from build123d import *

# Parameters (mm, degrees)
SKETCH_3_W          = 180
SKETCH_3_H          = 43
EXTRUDE_1_DEPTH     = 12
CUT_EXTRUDE_1_DEPTH = 52
CUT_EXTRUDE_2_DEPTH = 5
CUT_EXTRUDE_3_DEPTH = 5
SKETCH_8_W          = 55
SKETCH_8_H          = 37
CUT_EXTRUDE_4_DEPTH = 10.5
CUT_EXTRUDE_5_DEPTH = 3
SKETCH_10_W         = 62.128790526
SKETCH_10_H         = 8.683746703
CUT_EXTRUDE_6_DEPTH = 8
CUT_EXTRUDE_8_DEPTH = 9
FILLET_3_R          = 3
FILLET_4_R          = 2.5


with BuildPart() as part:
    # 草图3 → 凸台-拉伸1 (new body)
    with BuildSketch(Plane(origin=(0, 0, 0), x_dir=(1, 0, 0), z_dir=(0, 1, 0))):
        with Locations((50.068597249, 7.753123643)):
            Rectangle(SKETCH_3_W, SKETCH_3_H)
    extrude(amount=EXTRUDE_1_DEPTH)

    # 草图4 → 切除-拉伸1 (cut)
    with BuildSketch(Plane(origin=(0, 0, 0), x_dir=(1, 0, 0), z_dir=(0, 1, 0))):
        Polygon((-22.469613434, -5.858946979), (26.002261286, -5.858946979), (29.068597249, -13.746876357), (-25.931402751, -13.746876357), align=None)
    extrude(amount=CUT_EXTRUDE_1_DEPTH, mode=Mode.SUBTRACT)

    # 草图5 → 切除-拉伸2 (cut)
    with BuildSketch(Plane(origin=(0, 12, 0), x_dir=(1, 0, 0), z_dir=(0, 1, 0))):
        Polygon((140.068597249, 7.753123643), (140.068597249, 22.753123643), (125.276479966, 22.753123643), (125.276479966, -7.246876357), (140.068597249, -7.246876357), align=None)
    extrude(amount=-CUT_EXTRUDE_2_DEPTH, mode=Mode.SUBTRACT)

    # 草图7 → 切除-拉伸3 (cut)
    with BuildSketch(Plane(origin=(0, 12, 0), x_dir=(1, 0, 0), z_dir=(0, 1, 0))):
        Polygon((125.276479966, 7.753123643), (125.276479966, 25.753123643), (100.500825538, 25.753123643), (100.500825538, -10.246876357), (125.276479966, -10.246876357), align=None)
    extrude(amount=-CUT_EXTRUDE_3_DEPTH, mode=Mode.SUBTRACT)

    # 草图8 → 切除-拉伸4 (cut)
    with BuildSketch(Plane(origin=(0, 12, 0), x_dir=(1, 0, 0), z_dir=(0, 1, 0))):
        with Locations((63.776287419, 7.753123643)):
            Rectangle(SKETCH_8_W, SKETCH_8_H)
    extrude(amount=-CUT_EXTRUDE_4_DEPTH, mode=Mode.SUBTRACT)

    # 草图9 → 切除-拉伸5 (cut)
    with BuildSketch(Plane(origin=(0, 12, 0), x_dir=(1, 0, 0), z_dir=(0, 1, 0))):
        Polygon((91.276287419, 26.253123643), (96.635770173, 26.253123643), (96.635770173, 22.130591531), (96.635770173, 13.862098754), (97.813575381, 11.877191358), (100.500825538, 11.877191358), (100.500825538, 3.393971617), (96.236747254, 3.393971617), (92.132656028, 10.310430274), (92.132656028, 21.255120764), (91.276287419, 21.255120764), align=None)
    extrude(amount=-CUT_EXTRUDE_5_DEPTH, mode=Mode.SUBTRACT)

    # 草图10 → 切除-拉伸6 (cut)
    with BuildSketch(Plane(origin=(0, 12, 0), x_dir=(1, 0, 0), z_dir=(0, 1, 0))):
        with Locations((1.934159822, -6.405003006)):
            Rectangle(SKETCH_10_W, SKETCH_10_H)
    extrude(amount=-CUT_EXTRUDE_6_DEPTH, mode=Mode.SUBTRACT)

    # 草图11 → 切除-拉伸8 (cut)
    with BuildSketch(Plane(origin=(0, 12, 0), x_dir=(1, 0, 0), z_dir=(0, 1, 0))):
        Polygon((32.998555085, -10.746876357), (-36.5396752, -10.746876357), (-36.5396752, 26.253123643), (36.276287419, 26.253123643), (36.276287419, -2.167243749), (32.998555085, -2.063129654), align=None)
    extrude(amount=-CUT_EXTRUDE_8_DEPTH, mode=Mode.SUBTRACT)

    # 圆角3
    fillet_3_edges = [part.edges().sort_by_distance(p)[0] for p in [
        (-39.931402751, 6, -29.253123643),
        (140.068597249, 6, -29.253123643),
        (140.068597249, 6, 13.746876357),
        (-39.931402751, 6, 13.746876357),
    ]]
    fillet(fillet_3_edges, radius=FILLET_3_R)

    # 圆角4
    fillet_4_edges = [part.edges().sort_by_distance(p)[0] for p in [
        (83.068597249, 0, 13.746876357),
        (50.068597249, 0, -29.253123643),
        (-31.431402751, 0, 13.746876357),
        (-39.931402751, 0, -7.753123643),
        (140.068597249, 0, -7.753123643),
        (-39.052723094, 0, -28.374443987),
        (-39.052723094, 0, 12.8681967),
        (139.189917593, 0, 12.8681967),
        (139.189917593, 0, -28.374443987),
    ]]
    fillet(fillet_4_edges, radius=FILLET_4_R)


solid = part.part
Verification items for the finished model (mm, model axes). A direction names the side the tool comes from. Give positions to 0.01 mm unless a question says otherwise; leave off trailing zeros. Loops run counter-clockwise (first coordinate to the right, second up) from the corner with the lowest first, then second, coordinate; pieces in that order, holes last.
1) Depth check by flat-ended pin: pin 1 Ø8 at (x, z) = (25.5, 6) entering from -Y; pin 2 Ø1 at (x, y) = (22, 2.5) entering from +Z; pin 3 Ø5.5 at (y, z) = (10.5, -4.5) entering from +X; pin 4 Ø8 at (x, z) = (73.5, -13) entering from +Y. Enter the tip coordinate at first touch or a pass-through.
2) Sectioned sample at D-D, the plane x = -2.5. Enter the section's corners in (y, z).
3) Set-up check for faces 1 (the flat face through (28.195, 4.583, 11.501)), 2 (the flat face through (29, 7, -26.253)), 3 (the flat face through (94.213, 10.521, -6.804)): record each of +Z, -Z, +X, -X, +Y, -Y from which the full face is reachable in a straight line by a thin tool's end or side.
4) Sectioned sample at C-C, the plane x = 116.5. Enter the section's corners in (y, z), then the cut area to 3 significant figures.
5) Draft check along Z on faces 4 (the flat face through (125.276, 10, -24)), 5 (the cylindrical face through (-39.076, 7.316, -28.351)), 6 (the flat face through (23, 12, -27)). Enter one of: pulls with the +Z half, pulls with the -Z half, needs draft (parallel to the pull), parting line crosses it, or undercut.
6) Sectioned sample at A-A, the plane x = 81. Enter the section's corners in (y, z).
7) Sectioned sample at B-B, the plane z = -8. Enter the section's corners in (x, y), then the cut area to 3 significant figures.
8) Thickness scan on line 1 along X through (y, z) = (11, -24); line 2 along X through (y, z) = (7.25, 9.5); line 3 along X through (y, z) = (6.75, -19.5). Record the ranges inside material, lowest first.
Answers:
1. pin 1: stops at y = 0
1. pin 2: stops at z = 5.86
1. pin 3: stops at x = 100.5
1. pin 4: stops at y = 1.5
2. outline: (0, -26.75) arc R2.5 ccw to (2.5, -29.25) - (12, -29.25) - (12, -26.25) - (3, -26.25) - (3, 5.86) - (0, 5.86) - close
3. face 1: +Z, +Y, -Y
3. face 2: +Y
3. face 3: +X, +Y
4. outline: (0, -26.75) arc R2.5 ccw to (2.5, -29.25) - (12, -29.25) - (12, -25.75) - (7, -25.75) - (7, 10.25) - (12, 10.25) - (12, 13.75) - (2.5, 13.75) arc R2.5 ccw to (0, 11.25) - close
4. area: 333 mm2
5. face 4: undercut
5. face 5: pulls with the -Z half
5. face 6: needs draft
6. outline: (0, -26.75) arc R2.5 ccw to (2.5, -29.25) - (12, -29.25) - (12, -26.25) - (1.5, -26.25) - (1.5, 10.75) - (12, 10.75) - (12, 13.75) - (2.5, 13.75) arc R2.5 ccw to (0, 11.25) - close
7. outline: (-39.93, 2.5) arc R2.5 ccw to (-37.43, 0) - (137.57, 0) arc R2.5 ccw to (140.07, 2.5) - (140.07, 7) - (100.5, 7) - (100.5, 9) - (93.5, 9) - (93.5, 12) - (91.28, 12) - (91.28, 1.5) - (36.28, 1.5) - (36.28, 3) - (-36.54, 3) - (-36.54, 12) - (-39.93, 12) - close
7. area: 706 mm2
8. line 1: x = -39.93 to -36.54, 96.64 to 100.5, 125.28 to 140.07
8. line 2: x = -39.93 to -36.54, 33 to 36.28, 91.28 to 100.5, 125.28 to 140.07
8. line 3: x = -39.93 to -36.54, 91.28 to 140.07
